Design review of the part shown in the three views and the two pictorial views. Dimensions are in mm from the part's minimum x, y and z. Give positions to 0.01 mm unless a question says otherwise; leave off trailing zeros. Loops run counter-clockwise (first coordinate to the right, second up) from the corner with the lowest first, then second, coordinate; pieces in that order, holes last. Notation, with made-up numbers: (-34, 15) - (-9, 15) arc R23 cw to (-9, 31) - close; hole circle Ø10 at (23.25, -35.5). An arc over 180 degrees is marked (long way). Put each result on its own line as item: value. Start each with the question number.
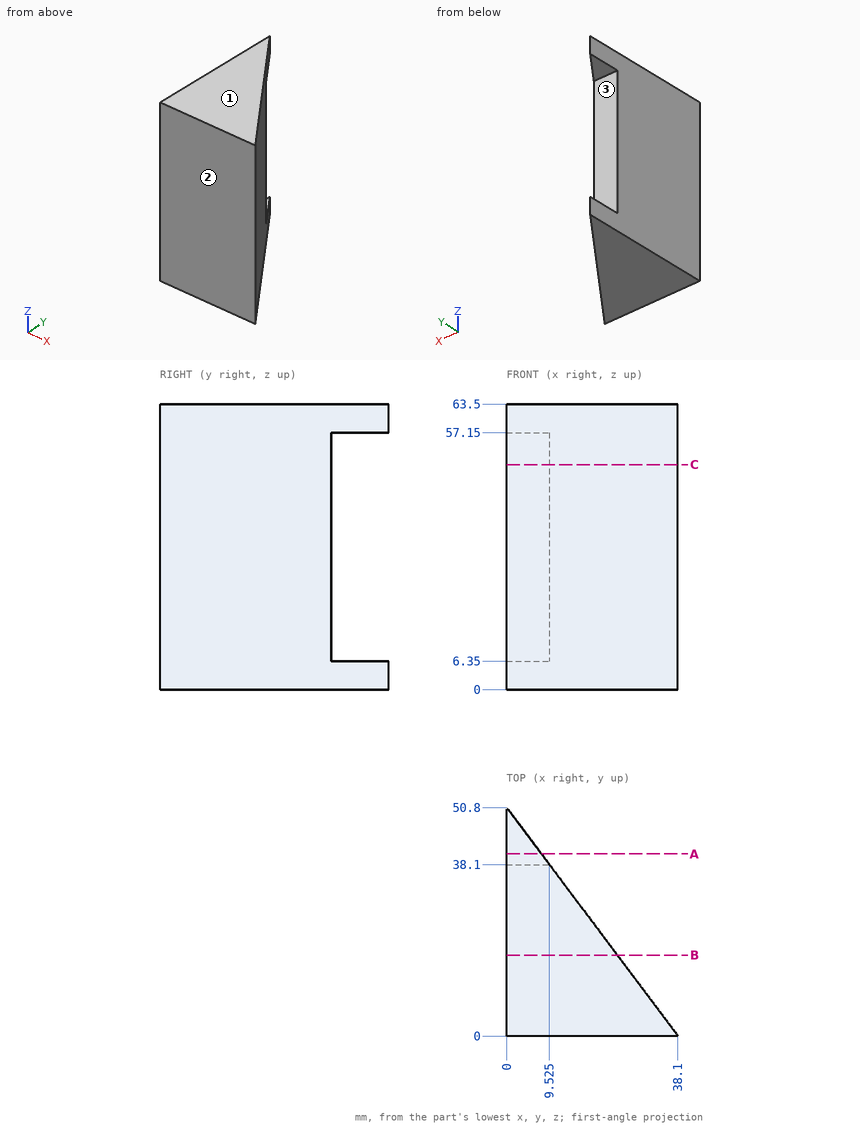
1) Wall thickness on probe 1 along Y at (x, z) = (9, 38.5); probe 2 along Y at (x, z) = (30, 30.5); probe 3 along X at (y, z) = (26, 30): over which ranges is each line inside the solid? List them lowest first.
2) Take a section at C-C on z = 50. State the section outline as (x, y) points (3 decimals), and give its area (3 significant figures).
3) Mouldability with a two-part tool opening along Z and no side actions: class the marked faces 1, 2 and 3 as released by +Z, released by -Z, zero draft, split by the parting line, or undercut.
4) Insertion check: P1, Ø4, axis at x = 23, z = 23, coming from the +Y side; P2, Ø4, axis at y = 8.5, z = 54, coming from the +X side (3 decimals); P3, Ø1.5, axis at x = 28, z = 30.5, coming from the +Y side. Each pin has a flat end and moves straight along its axis. Give the tip position at first contact, or say it passes through.
5) Take a section at B-B on y = 18. State the section outline as (x, z) points, and give its area (3 significant figures).
6) Take a section at A-A on y = 40.5. State the section outline as (x, z) points (3 decimals), and give its area (3 significant figures).
Answers follow:
1. probe 1: 0 to 38.1
1. probe 2: 0 to 10.8
1. probe 3: 0 to 18.6
2. outline: (0, 0) - (38.1, 0) - (9.525, 38.1) - (0, 38.1) - close
2. area: 907 mm2
3. face 1: released by +Z
3. face 2: zero draft
3. face 3: undercut
4. P1: y = 22.8
4. P2: x = 33.225
4. P3: y = 14.47
5. outline: (0, 0) - (24.6, 0) - (24.6, 63.5) - (0, 63.5) - close
5. area: 1,560 mm2
6. outline: (0, 0) - (7.725, 0) - (7.725, 6.35) - (0, 6.35) - close; (0, 57.15) - (7.725, 57.15) - (7.725, 63.5) - (0, 63.5) - close
6. area: 98.1 mm2
